Geometry check sheet. Reference: the model listing, model coordinates, mm. A direction names the side the tool comes from. Coordinates: 2 decimals unless noted, no trailing zeros. Write each loop counter-clockwise with the first axis right and the second up, starting at its lowest first coordinate (ties: lowest second). Pieces come first, ordered by that corner, then holes. Notation, with made-up numbers: (23.5, 10.5) -> (76.5, 10.5) arc R26 ccw to (76.5, 47.5) -> close; hole circle Ø7 at (37, 26). An arc over 180 degrees is marked (long way). Answer as CSV lines item,"result".
```python
from build123d import *

# Parameters (mm, degrees)
SKETCH1_R           = 12.7
SKETCH1_R_2         = 8.89
BOSS_EXTRUDE1_DEPTH = 16.7132
SKETCH1_3_R         = 8.89
BOSS_EXTRUDE2_DEPTH = 15.1511


with BuildPart() as part:
    # Sketch1 → Boss-Extrude1 (new body)
    with BuildSketch(Plane(origin=(0, 0, 0), x_dir=(1, 0, 0), z_dir=(0, 1, 0))):
        Circle(SKETCH1_R)
        Circle(SKETCH1_R_2, mode=Mode.SUBTRACT)
    extrude(amount=BOSS_EXTRUDE1_DEPTH)

    # Sketch1_3 → Boss-Extrude2 (add)
    with BuildSketch(Plane(origin=(0, 0, 0), x_dir=(1, 0, 0), z_dir=(0, 1, 0))):
        Circle(SKETCH1_3_R)
        Polygon((6.35, -3.666174209), (6.35, 3.666174209), (0, 7.332348419), (-6.35, 3.666174209), (-6.35, -3.666174209), (0, -7.332348419), align=None, mode=Mode.SUBTRACT)
    extrude(amount=BOSS_EXTRUDE2_DEPTH)


solid = part.part
```
Item 1: Cross-section at C-C, the plane x = -2.25. Record the cut outline in (y, z).
Responses:
outline,"(0, -12.5) -> (16.71, -12.5) -> (16.71, -8.6) -> (15.15, -8.6) -> (15.15, -6.03) -> (0, -6.03) -> close; (0, 6.03) -> (15.15, 6.03) -> (15.15, 8.6) -> (16.71, 8.6) -> (16.71, 12.5) -> (0, 12.5) -> close"
Item 2: Cross-section at D-D, the plane y = 15.5. Record the cut outline in (x, z).
Responses:
outline,"circle Ø25.4 at (0, 0); hole circle Ø17.78 at (0, 0)"
Item 3: Cross-section at B-B, the plane y = 1.75. Record the cut outline in (x, z), plus the area to 3 significant figures.
Responses:
outline,"circle Ø25.4 at (0, 0); hole (-6.35, -3.67) -> (0, -7.33) -> (6.35, -3.67) -> (6.35, 3.67) -> (0, 7.33) -> (-6.35, 3.67) -> close"
area,"367 mm2"
Item 4: Thickness scan on probe 1 along Z at (x, y) = (0, 16.25); probe 2 along X at (y, z) = (1, 0.25). Record the ranges inside material, lowest first.
Responses:
probe 1,"z = -12.7 to -8.89, 8.89 to 12.7"
probe 2,"x = -12.7 to -6.35, 6.35 to 12.7"
Item 5: Cross-section at A-A, the plane z = 0. Record the cut outline in (x, y).
Responses:
outline,"(-12.7, 0) -> (-6.35, 0) -> (-6.35, 15.15) -> (-8.89, 15.15) -> (-8.89, 16.71) -> (-12.7, 16.71) -> close; (6.35, 0) -> (12.7, 0) -> (12.7, 16.71) -> (8.89, 16.71) -> (8.89, 15.15) -> (6.35, 15.15) -> close"
Item 6: Release check for a two-part mould opening along Z. For faces 1 (the cylindrical face through (-2.75, 8.24, 12.4)), 2 (the flat face through (3.131, 7.469, 5.525)), 3 (the flat face through (-9, 16.713, 3)), 4 (the flat face through (-3.131, 7.469, -5.525)) record: +Z half, -Z half, draft (parallel to the pull), parting line (faces both ways), or undercut.
Responses:
face 1,"parting line"
face 2,"undercut"
face 3,"draft"
face 4,"undercut"
Item 7: Set-up check for faces 5 (the cylindrical face through (-1.93, 15.92, 8.68)), 6 (the flat face through (3.219, 7.469, -5.474)), 7 (the flat face through (3, 0, -6)): record each of +Z, -Z, +X, -X, +Y, -Y from which the full face is reachable in a straight line by a thin tool's end or side.
Responses:
face 5,"+Y"
face 6,"+Y, -Y"
face 7,"+Z, -Z, +X, -X, -Y"
Item 8: Depth check by flat-ended pin: pin 1 Ø5 at (x, y) = (7.5, 14.5) entering from -Z; pin 2 Ø4 at (y, z) = (10.5, 3) entering from -X; pin 3 Ø6 at (y, z) = (12.5, -9) entering from -X. Enter the tip coordinate at first touch or a pass-through.
Responses:
pin 1,"stops at z = -11.67"
pin 2,"stops at x = -12.66"
pin 3,"stops at x = -11.19"
